For this review, use the dimensioned drawing (mm, ordinates from the lowest corner) and the shaded views. Give positions to 0.01 mm unless a question says otherwise; leave off trailing zeros. Write each loop counter-clockwise with the first axis right and the second up, starting at its lowest first coordinate (ties: lowest second). Pieces come first, ordered by that corner, then holes. Notation, with made-up numbers: (3, 86) -> (17, 86) arc R12 cw to (17, 95) -> close; hole circle Ø6 at (6.25, -32). An arc over 180 degrees is marked (long way). Write each question's results on one line, items separated by ' | '. Start each with the question number.
(1) Take a section at D-D (z = 2.75). State the section outline as (x, y) points.
(2) Mouldability with a two-part tool opening along X and no side actions: class the marked faces 1, 2, 3 and 4 as released by +X, released by -X, zero draft, split by the parting line, or undercut.
(3) Take a section at C-C (y = 31.5). State the section outline as (x, z) points.
(4) Take a section at B-B (z = 5.75). State the section outline as (x, y) points, plus the area to 3 significant figures.
(5) Clearance check with flat-ended pins moving along their axes: pin 1 (5 mm diameter, centred on x = 9, y = 7, fed in from -Z); pin 2 (12 mm diameter, centred on x = 29, y = 9.5, fed in from -Z). State where each tip first meets the part, or that it passes through.
(6) Take a section at A-A (x = 34). State the section outline as (y, z) points.
(7) To check wall thickness, follow probe 1 along Y at (x, z) = (9, 6.5); probe 2 along Z at (x, y) = (6, 11); probe 3 along X at (y, z) = (52.5, 6). State the ranges of each line that lie inside material, in increasing order.
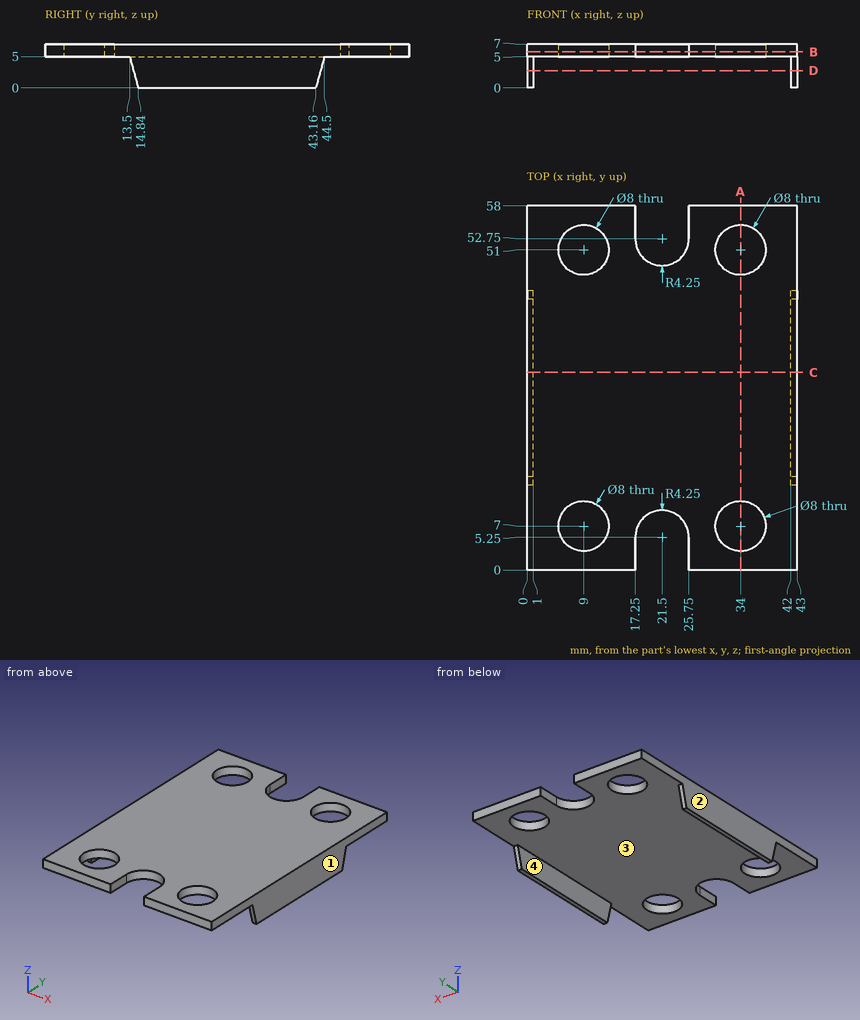
Report:
1) outline: (0, 14.1) -> (1, 14.1) -> (1, 43.9) -> (0, 43.9) -> close; (42, 14.1) -> (43, 14.1) -> (43, 43.9) -> (42, 43.9) -> close
2) face 1: released by +X | face 2: released by -X | face 3: undercut | face 4: undercut
3) outline: (0, 0) -> (1, 0) -> (1, 5) -> (42, 5) -> (42, 0) -> (43, 0) -> (43, 7) -> (0, 7) -> close
4) outline: (0, 0) -> (17.25, 0) -> (17.25, 5.25) arc R4.25 cw to (25.75, 5.25) -> (25.75, 0) -> (43, 0) -> (43, 58) -> (25.75, 58) -> (25.75, 52.75) arc R4.25 cw to (17.25, 52.75) -> (17.25, 58) -> (0, 58) -> close; hole circle Ø8 at (9, 7); hole circle Ø8 at (9, 51); hole circle Ø8 at (34, 7); hole circle Ø8 at (34, 51) | area: 2,150 mm2
5) pin 1: through | pin 2: z = 5
6) outline: (0, 5) -> (3, 5) -> (3, 7) -> (0, 7) -> close; (11, 5) -> (47, 5) -> (47, 7) -> (11, 7) -> close; (55, 5) -> (58, 5) -> (58, 7) -> (55, 7) -> close
7) probe 1: 0 to 3, 11 to 47, 55 to 58 | probe 2: 5 to 7 | probe 3: 0 to 5.29, 12.71 to 17.26, 25.74 to 30.29, 37.71 to 43
